The model under review builds one solid part; all positions refer to its coordinate system, in mm. A direction names the side the tool comes from. Coordinates: 2 decimals unless noted, no trailing zeros. Order: outer loops, then holes, each group sorted by start corner. A loop starts at its lowest first (then second) coordinate and runs counter-clockwise, first axis right, second up. Notation, with made-up numbers: (-16.5, 45.25) - (38.5, 45.25) arc R30 ccw to (38.5, 68.25) - close; hole circle Ø1 at (54.25, 57.5). An arc over 180 degrees is marked (long way). Answer in a Markdown table with one row per item.
```python
from build123d import *

# Parameters (mm, degrees)
EXTRUDE_1_DEPTH     = 10
SKETCH_2_W          = 10
SKETCH_2_H          = 20
EXTRUDE_2_DEPTH     = 30
CUT_EXTRUDE_1_DEPTH = 30


with BuildPart() as part:
    # 草圖1 → 填料-伸長1 (new body)
    with BuildSketch(Plane(origin=(0, 0, 0), x_dir=(1, 0, 0), z_dir=(0, 1, 0))):
        with BuildLine():
            Line((0, 10), (0, 0))
            Line((0, 0), (-10, 0))
            Line((-10, 0), (-10, -20))
            ThreePointArc((-10, -20), (-8.739957075, -19.920296963), (-7.5, -19.682458366))
            ThreePointArc((-7.5, -19.682458366), (-7.410977969, -19.841638388), (-7.320508076, -20))
            Line((-7.320508076, -20), (10, -20))
            Line((10, -20), (10, 10))
            Line((10, 10), (0, 10))
        make_face()
        with BuildLine():
            Line((-10, -20), (-10, 0))
            ThreePointArc((-10, 0), (-20, -10), (-10, -20))
        make_face()
        with BuildLine():
            Line((10, -20), (10, -30))
            ThreePointArc((10, -30), (30, -10), (10, 10))
            Line((10, 10), (10, -20))
        make_face()
    extrude(amount=EXTRUDE_1_DEPTH)

    # 草圖2 → 填料-伸長2 (add)
    with BuildSketch(Plane.XZ):
        with Locations((-5, -10)):
            Rectangle(SKETCH_2_W, SKETCH_2_H)
    extrude(amount=-EXTRUDE_2_DEPTH)

    # 草圖3 → 除料-伸長1 (cut)
    with BuildSketch(Plane(origin=(0, 0, 0), x_dir=(0, 0, -1), z_dir=(1, 0, 0))):
        Polygon((20, 30), (0, 10), (0, 30), align=None)
    extrude(amount=-CUT_EXTRUDE_1_DEPTH, mode=Mode.SUBTRACT)


solid = part.part
```
Item 1: To check wall thickness, follow line 1 (X direction, y = 16.75, z = -13.5); line 2 (Y direction, x = -14, z = 15.5); line 3 (Z direction, x = 1, y = 9.75). State the ranges of each line that lie inside material, in increasing order. Write a range as from..to.
Check values:
| item | result |
|---|---|
| line 1 | -10..0 |
| line 2 | 0..10 |
| line 3 | -10..20 |
Item 2: We need section B-B, the plane y = 3. Write out the cut boundary in (x, z).
Check values:
| item | result |
|---|---|
| outline | (-10, -20) - (0, -20) - (0, -10) - (10, -10) arc R20 ccw to (10, 30) - (10, 20) - (-7.32, 20) arc R20 ccw to (-7.5, 19.68) arc R10 ccw (long way) to (-10, 0) - close |
Item 3: Clearance check with flat-ended pins moving along their axes: pin 1 Ø1.5 at (y, z) = (4.5, 5) entering from -X; pin 2 Ø11 at (x, y) = (6.5, 4.5) entering from -Z; pin 3 Ø5 at (y, z) = (6.5, 25.5) entering from -X. State where each tip first meets the part, or that it passes through.
Check values:
| item | result |
|---|---|
| pin 1 | x = -19.05 |
| pin 2 | z = -10 |
| pin 3 | x = 10 |
Item 4: We need section C-C, the plane x = -2. Write out the cut boundary in (y, z), then the cut area to 3 significant figures.
Check values:
| item | result |
|---|---|
| outline | (0, -20) - (30, -20) - (10, 0) - (10, 20) - (0, 20) - close |
| area | 600 mm^2 |
Item 5: We need section A-A, the plane z = -6. Write out the cut boundary in (x, y), then the cut area to 3 significant figures.
Check values:
| item | result |
|---|---|
| outline | (-10, 0) - (22, 0) - (22, 10) - (0, 10) - (0, 16) - (-10, 16) - close |
| area | 380 mm^2 |
Item 6: Tool access review of faces 1 (the face through (10, 5, 25)), 2 (the face through (5, 10, 10)), 3 (the face through (-10, 11, -12)), 4 (the face through (-5, 15, -20)), 5 (the face through (5, 5, -10)): name each direction out of +Z, -Z, +X, -X, +Y, -Y from which nothing blocks a thin tool from reaching the whole face with its end or side.
Check values:
| item | result |
|---|---|
| face 1 | +Z, -X, +Y, -Y |
| face 2 | +Z, +X, +Y |
| face 3 | -Z, -X, +Y, -Y |
| face 4 | -Z, +X, -X, +Y, -Y |
| face 5 | -Z, +X, +Y, -Y |
Item 7: We need section D-D, the plane z = 10. Write out the cut boundary in (x, y).
Check values:
| item | result |
|---|---|
| outline | (-20, 0) - (30, 0) - (30, 10) - (-20, 10) - close |
